Design review of the part built by this model. Coordinates are the model's own, in mm. A direction names the side the tool comes from. Coordinates: 2 decimals unless noted, no trailing zeros. Loops run counter-clockwise (first coordinate to the right, second up) from the corner with the lowest first, then second, coordinate; pieces in that order, holes last.
Q1. Add section D-D on x = 16. Give the boundary of the cut face in (y, z), and give its area (3 significant figures).
Q2. Add section B-B on z = 0. Give the boundary of the cut face in (x, y).
Q3. Add section A-A on x = 0. Give the boundary of the cut face in (y, z), and give its area (3 significant figures).
Q4. Machinability: for faces 1 (the face through (0.88, -6.35, -11.23)), 2 (the face through (18.737, -3.913, 18.705)), which of the approach directions +Z, -Z, +X, -X, +Y, -Y give a long, thin tool a straight path to every point of the face, cutting with its end or side? Answer none if there is none.
Q5. Wall thickness on probe 1 along X at (y, z) = (-2.5, -15); probe 2 along X at (y, z) = (-7, 14); probe 3 along Z at (x, y) = (13, -5): over which ranges is each line inside the solid? List them lowest first.
Q6. Add section C-C on y = -5.75. Give the boundary of the cut face in (x, z) (3 decimals).
Q7. Draft analysis for pull direction Z (two halves, no side actions). For faces 3 (the face through (0, -4, -19.844)), 4 (the face through (10.6, -7.13, 3.34)), 5 (the face through (14.393, -3.913, 11.982)), 6 (the face through (-19.844, -4, 0)), state which applies: released by +Z, released by -Z, zero draft, split by the parting line, or undercut.
```python
from build123d import *

# Parameters (mm, degrees)
F0_W     = 39.6875
F0_H     = 39.6875
F0_R     = 3.175
F0_R_2   = 12.7
F0_R_3   = 11.1125
F1_DEPTH = 7.9375
F2_DEPTH = 6.35
F3_SIZE  = 2.245403


with BuildPart() as f1:
    # F0 (on Front) → F1 (new body)
    with BuildSketch(Plane.XZ):
        Rectangle(F0_W, F0_H)
        with Locations((-15.08125, -15.08125)):
            Circle(F0_R, mode=Mode.SUBTRACT)
        with Locations((15.08125, -15.08125)):
            Circle(F0_R, mode=Mode.SUBTRACT)
        with Locations((-15.08125, 15.08125)):
            Circle(F0_R, mode=Mode.SUBTRACT)
        Circle(F0_R_2, mode=Mode.SUBTRACT)
        with Locations((15.08125, 15.08125)):
            Circle(F0_R, mode=Mode.SUBTRACT)
        Circle(F0_R_2)
        Circle(F0_R_3, mode=Mode.SUBTRACT)
    extrude(amount=F1_DEPTH)

    # F0 (on Front) → F2 (cut)
    with BuildSketch(Plane.XZ):
        Circle(F0_R_2)
        Circle(F0_R_3, mode=Mode.SUBTRACT)
    extrude(amount=F2_DEPTH, mode=Mode.SUBTRACT)

    # F3
    f3_edges = [f1.edges().sort_by_distance(p)[0] for p in [
        (19.84375, -3.96875, 19.84375),
        (19.84375, -3.96875, -19.84375),
        (-19.84375, -3.96875, -19.84375),
        (-19.84375, -3.96875, 19.84375),
    ]]
    chamfer(f3_edges, length=F3_SIZE)


solid = f1.part
```
Entries:
1. outline: (-7.94, -19.84) - (0, -19.84) - (0, -18.12) - (-7.94, -18.12) - close; (-7.94, -12.04) - (0, -12.04) - (0, 12.04) - (-7.94, 12.04) - close; (-7.94, 18.12) - (0, 18.12) - (0, 19.84) - (-7.94, 19.84) - close
1. area: 219 mm2
2. outline: (-19.84, -7.94) - (-11.11, -7.94) - (-11.11, -6.35) - (-12.7, -6.35) - (-12.7, 0) - (-19.84, 0) - close; (11.11, -7.94) - (19.84, -7.94) - (19.84, 0) - (12.7, 0) - (12.7, -6.35) - (11.11, -6.35) - close
3. outline: (-7.94, -19.84) - (0, -19.84) - (0, -12.7) - (-6.35, -12.7) - (-6.35, -11.11) - (-7.94, -11.11) - close; (-7.94, 11.11) - (-6.35, 11.11) - (-6.35, 12.7) - (0, 12.7) - (0, 19.84) - (-7.94, 19.84) - close
3. area: 118 mm2
4. face 1: +Y
4. face 2: +Z, +X, +Y, -Y
5. probe 1: x = -19.84 to -18.26, -11.91 to 11.91, 18.26 to 19.84
5. probe 2: x = -19.84 to -18.07, -12.1 to 12.1, 18.07 to 19.84
5. probe 3: z = -19.84 to -17.48, -12.68 to 12.68, 17.48 to 19.84
6. outline: (-19.844, -17.598) - (-17.598, -19.844) - (17.598, -19.844) - (19.844, -17.598) - (19.844, 17.598) - (17.598, 19.844) - (-17.598, 19.844) - (-19.844, 17.598) - close; hole circle Ø6.35 at (-15.081, -15.081); hole circle Ø6.35 at (-15.081, 15.081); hole circle Ø25.4 at (0, 0); hole circle Ø6.35 at (15.081, -15.081); hole circle Ø6.35 at (15.081, 15.081)
7. face 3: released by -Z
7. face 4: undercut
7. face 5: undercut
7. face 6: zero draft
